Could you check a few things on this model? Use its own coordinates, in mm. Face numbers are marked on the shaded views. A direction names the side the tool comes from. Coordinates: 2 decimals unless noted, no trailing zeros. Order: outer loops, then holes, each group sorted by start corner. A loop starts at its lowest first (then second) coordinate and runs counter-clockwise, first axis right, second up. Notation, with made-up numbers: (-6.75, -35) -> (20.25, -35) arc R20 ccw to (20.25, 0) -> close; hole circle Ø8 at (68.5, 33). An arc over 180 degrees is marked (long way). Use a Markdown table: item, result. Add a question column.
1) Which directions (+Z, -Z, +X, -X, +Y, -Y) give clear straight access to the entire face, cutting with the end or side of a thin tool? Please do the marked faces 1, 2 and 3.
2) If we section it at A-A (y = 0): Write out the boundary of the cut face in (x, z).
3) If we section it at B-B (x = 4): Write out the boundary of the cut face in (y, z), plus the area to 3 significant figures.
4) Will these pins go through, and if not, where does the flat tip stop? pin 1 Ø6 at (x, y) = (-14, 20) entering from -Z; pin 2 Ø1 at (x, z) = (3, 4) entering from +Y; pin 3 Ø1.5 at (y, z) = (6, -1.5) entering from +X; pin 4 Ø6 at (x, z) = (-19, 2) entering from -Y.
5) If I drill on L1, parallel to Y at x = -22.5, z = 0.8; L2, parallel to Y at x = 23, z = 0.75; L3, parallel to X at y = -10, z = 3.5, over which ranges is the centre line in solid material (lowest first)? Write a range as [from, to].
6) If we section it at D-D (x = -14): Write out the boundary of the cut face in (y, z), plus the area to 3 significant figures.
7) If we section it at C-C (z = 4.25): Write out the boundary of the cut face in (x, y).
```python
from build123d import *

# Parameters (mm, degrees)
SKETCH1_W                    = 50
SKETCH1_H                    = 50
BOSS_EXTRUDE1_DEPTH          = 1.5
SKETCH2_W                    = 35
SKETCH2_H                    = 35
BOSS_EXTRUDE2_DEPTH          = 4
SKETCH3_W                    = 32
SKETCH3_H                    = 32
BOSS_EXTRUDE3_DEPTH          = 0.1
F_3_0_3_DIAMETER_HOLE1_D     = 3
F_4_0_4_DIAMETER_HOLE1_D     = 4
F_4_0_4_DIAMETER_HOLE1_DEPTH = 0.1
FILLET1_R                    = 2.5
CHAMFER1_SIZE                = 5.656854249
CHAMFER2_SIZE                = 0.5
SKETCH8_W                    = 30
SKETCH8_H                    = 30
BOSS_EXTRUDE4_DEPTH          = 5


with BuildPart() as part:
    # Sketch1 → Boss-Extrude1 (new body)
    with BuildSketch(Plane.XY.offset(1.5)):
        Rectangle(SKETCH1_W, SKETCH1_H)
    extrude(amount=-BOSS_EXTRUDE1_DEPTH)

    # Sketch2 → Boss-Extrude2 (add)
    with BuildSketch(Plane.XY.offset(1.5)):
        Rectangle(SKETCH2_W, SKETCH2_H)
    extrude(amount=BOSS_EXTRUDE2_DEPTH)

    # Sketch3 → Boss-Extrude3 (add)
    with BuildSketch(Plane.XY.offset(5.5)):
        Rectangle(SKETCH3_W, SKETCH3_H)
    extrude(amount=BOSS_EXTRUDE3_DEPTH)

    # Ø3.0 (3) Diameter Hole1 (through all)
    with Locations(Plane.XY.offset(1.5)):
        with Locations((22.5, -22.5), (-22.5, 22.5), (22.5, 22.5), (-22.5, -22.5)):
            Hole(F_3_0_3_DIAMETER_HOLE1_D / 2)

    # Ø4.0 (4) Diameter Hole1
    with Locations(Plane.XY.offset(5.6)):
        with Locations((0, -4)):
            Hole(F_4_0_4_DIAMETER_HOLE1_D / 2, depth=F_4_0_4_DIAMETER_HOLE1_DEPTH)

    # Fillet1
    fillet1_edges = [part.edges().sort_by_distance(p)[0] for p in [
        (-17.5, 17.5, 3.5),
        (-17.5, -17.5, 3.5),
        (17.5, -17.5, 3.5),
        (17.5, 17.5, 3.5),
        (25, -25, 0.75),
        (-25, -25, 0.75),
        (-25, 25, 0.75),
        (25, 25, 0.75),
    ]]
    fillet(fillet1_edges, radius=FILLET1_R)

    # Chamfer1
    chamfer1_edges = [part.edges().sort_by_distance(p)[0] for p in [
        (16, 16, 5.55),
        (-16, -16, 5.55),
    ]]
    chamfer(chamfer1_edges, length=CHAMFER1_SIZE)

    # Chamfer2
    chamfer2_edges = [part.edges().sort_by_distance(p)[0] for p in [
        (17.5, 0, 5.5),
        (0, -17.5, 5.5),
        (-17.5, 0, 5.5),
        (0, 17.5, 5.5),
        (-16.767766953, 16.767766953, 5.5),
        (-16.767766953, -16.767766953, 5.5),
        (16.767766953, 16.767766953, 5.5),
        (16.767766953, -16.767766953, 5.5),
    ]]
    chamfer(chamfer2_edges, length=CHAMFER2_SIZE)

    # Sketch8 → Boss-Extrude4 (add)
    with BuildSketch(Plane(origin=(0, 0, 0), x_dir=(-1, 0, 0), z_dir=(0, 0, -1))):
        with Locations((10, 0.618109873)):
            Rectangle(SKETCH8_W, SKETCH8_H)
    extrude(amount=BOSS_EXTRUDE4_DEPTH)


solid = part.part
```
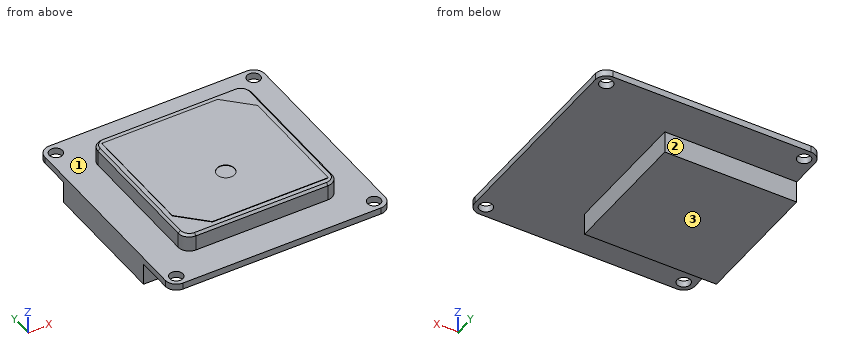
Answer sheet:
| question | item | result |
|---|---|---|
| 1 | face 1 | +Z |
| 1 | face 2 | -Z, +X, -X, +Y |
| 1 | face 3 | -Z, +X, -X, +Y, -Y |
| 2 | outline | (-25, -5) -> (5, -5) -> (5, 0) -> (25, 0) -> (25, 1.5) -> (17.5, 1.5) -> (17.5, 5) -> (17, 5.5) -> (16, 5.5) -> (16, 5.6) -> (-16, 5.6) -> (-16, 5.5) -> (-17, 5.5) -> (-17.5, 5) -> (-17.5, 1.5) -> (-25, 1.5) -> close |
| 3 | outline | (-25, 0) -> (-14.38, 0) -> (-14.38, -5) -> (15.62, -5) -> (15.62, 0) -> (25, 0) -> (25, 1.5) -> (17.5, 1.5) -> (17.5, 5) -> (17, 5.5) -> (16, 5.5) -> (16, 5.6) -> (-16, 5.6) -> (-16, 5.5) -> (-17, 5.5) -> (-17.5, 5) -> (-17.5, 1.5) -> (-25, 1.5) -> close |
| 3 | area | 368 mm2 |
| 4 | pin 1 | z = 0 |
| 4 | pin 2 | y = 17.5 |
| 4 | pin 3 | x = 5 |
| 4 | pin 4 | y = -25 |
| 5 | L1 | [-25, -24], [-21, 21], [24, 25] |
| 5 | L2 | [-24.95, -23.91], [-21.09, 21.09], [23.91, 24.95] |
| 5 | L3 | [-17.5, 17.5] |
| 6 | outline | (-25, 0) -> (-14.38, 0) -> (-14.38, -5) -> (15.62, -5) -> (15.62, 0) -> (25, 0) -> (25, 1.5) -> (17.5, 1.5) -> (17.5, 5) -> (17, 5.5) -> (16, 5.5) -> (16, 5.6) -> (-12.34, 5.6) -> (-12.34, 5.5) -> (-17, 5.5) -> (-17.5, 5) -> (-17.5, 1.5) -> (-25, 1.5) -> close |
| 6 | area | 368 mm2 |
| 7 | outline | (-17.5, -15) arc R2.5 ccw to (-15, -17.5) -> (15, -17.5) arc R2.5 ccw to (17.5, -15) -> (17.5, 15) arc R2.5 ccw to (15, 17.5) -> (-15, 17.5) arc R2.5 ccw to (-17.5, 15) -> close |
